from build123d import *

# Parameters (mm, degrees)
BOSS_EXTRUDE2_DEPTH   = 10
BOSS_EXTRUDE2_2_DEPTH = 10
SKETCH4_R             = 2.5
BOSS_EXTRUDE3_DEPTH   = 10
SKETCH8_R             = 22.839298689
CUT_EXTRUDE1_DEPTH    = 10


with BuildPart() as part:
    # Sketch1 → Boss-Extrude2 (new body)
    with BuildSketch(Plane(origin=(0, 0, 0), x_dir=(1, 0, 0), z_dir=(0, 1, 0))):
        Polygon((-26.25, 10.75), (-15, 10.75), (-15, 0), (-23.984756923, -9), (-26.25, -9), (-26.25, -0.114272299), (-29.438415679, -2.555067389), (-29.438415679, 11.073293435), (-26.25, 9.911985917), align=None)
    extrude(amount=BOSS_EXTRUDE2_DEPTH)

    # Sketch8 → Cut-Extrude1 (cut)
    with BuildSketch(Plane(origin=(0, 0, 0), x_dir=(1, 0, 0), z_dir=(0, 1, 0))):
        with Locations((-20.905433381, 4.192616326)):
            Circle(SKETCH8_R)
    extrude(amount=CUT_EXTRUDE1_DEPTH, mode=Mode.SUBTRACT)


with BuildPart() as body_2:
    # Sketch1 → Boss-Extrude2 2 (new body)
    with BuildSketch(Plane(origin=(0, 0, 0), x_dir=(1, 0, 0), z_dir=(0, 1, 0))):
        Polygon((26.25, 10.75), (26.25, 9.911985917), (29.438415679, 11.073293435), (29.438415679, -2.555067389), (26.25, -0.114272299), (26.25, -9), (23.984756923, -9), (15, 0), (15, 10.75), align=None)
    extrude(amount=BOSS_EXTRUDE2_2_DEPTH)

    # Sketch4 → Boss-Extrude3 (add)
    with BuildSketch(Plane(origin=(0, 0, 0), x_dir=(1, 0, 0), z_dir=(0, 1, 0))):
        with BuildLine():
            Line((28.75, -9.5), (33.5, -9.5))
            Line((33.5, -9.5), (33.5, 22.996479512))
            Line((33.5, 22.996479512), (40.345191882, 53.478179684))
            ThreePointArc((40.345191882, 53.478179684), (42.346706654, 60.478565285), (47.83611753, 65.261642557))
            ThreePointArc((47.83611753, 65.261642557), (56.530633029, 70.937419635), (48.815741717, 77.886484122))
            ThreePointArc((48.815741717, 77.886484122), (31.869937483, 69.990732218), (13.180106847, 70.430516322))
            ThreePointArc((13.180106847, 70.430516322), (7.243272391, 73.413222616), (0.765261217, 74.88899747))
            ThreePointArc((0.765261217, 74.88899747), (-7.423605548, 67.770164785), (0.226137573, 60.074922886))
            ThreePointArc((0.226137573, 60.074922886), (22.453224616, 50.257390562), (28.75, 26.78873148))
            Line((28.75, 26.78873148), (28.75, -9.5))
        make_face()
        with Locations(Location((0, 67.5, 0), (0, 0, 270))):
            Circle(SKETCH4_R, mode=Mode.SUBTRACT)
        with Locations(Location((50, 71.444163901, 0), (0, 0, 270))):
            Circle(SKETCH4_R, mode=Mode.SUBTRACT)
    extrude(amount=BOSS_EXTRUDE3_DEPTH)


solid = body_2.part
The model under review builds one solid part; all positions refer to its coordinate system, in mm. A direction names the side the tool comes from. Give positions to 0.01 mm unless a question says otherwise; leave off trailing zeros. Loops run counter-clockwise (first coordinate to the right, second up) from the corner with the lowest first, then second, coordinate; pieces in that order, holes last. Notation, with made-up numbers: (-28, 1.5) -> (-13, 1.5) arc R12 ccw to (-13, 9.5) -> close; hole circle Ø3 at (70.25, -22). An arc over 180 degrees is marked (long way). Put each result on its own line as item: value. Start each with the question number.
1. For faces 5 (the face through (7.33, 4.93, -73.38)), 6 (the face through (26.25, 5, 4)), 7 (the face through (25, 5, 9)), 8 (the face through (33.5, 5, -7)), list the 3-axis set-ups (+Z, -Z, +X, -X, +Y, -Y) from which the entire face can be reached by the end or side of a thin tool; tool diameter is ignored.
2. We need section D-D on z = -2. State the section outline as (x, y) points, then the cut area to 3 significant figures.
3. We need section B-B on z = -67.5. State the section outline as (x, y) points.
4. Clearance check with flat-ended pins moving along their axes: P1, Ø6, axis at x = 41.5, y = 4, coming from the -Z side; P2, Ø4, axis at x = 50, z = -71.44, coming from the -Y side; P3, Ø3, axis at y = 6, z = -16, coming from the -X side; P4, Ø3, axis at y = 4.5, z = -4, coming from the -X side. State where each tip first meets the part, or that it passes through.
5. We need section A-A on x = 50. State the section outline as (y, z) points.
6. Wall thickness on probe 1 along X at (y, z) = (2.25, -14); probe 2 along X at (y, z) = (5.5, -67.5); probe 3 along Z at (x, y) = (18, 2.75): over which ranges is each line inside the solid? List them lowest first.
7. We need section C-C on y = 5.5. State the section outline as (x, z) points, then the cut area to 3 significant figures.
8. Mouldability with a two-part tool opening along Z and no side actions: class faces 1 (the face through (21, 5, -10.75)), 2 (the face through (31, 5, 9.5)), 3 (the face through (0.751, 4.93, -65.115)), 4 (the face through (27, 0, -47)) as released by +Z, released by -Z, zero draft, split by the parting line, or undercut.
Determined:
1. face 5: -Z, +Y, -Y
1. face 6: +Z, +Y, -Y
1. face 7: +Z, -X, +Y, -Y
1. face 8: +Z, +X, +Y, -Y
2. outline: (15, 0) -> (33.5, 0) -> (33.5, 10) -> (15, 10) -> close
2. area: 185 mm^2
3. outline: (-7.43, 0) -> (-2.5, 0) -> (-2.5, 10) -> (-7.43, 10) -> close; (2.5, 0) -> (55.23, 0) -> (55.23, 10) -> (2.5, 10) -> close
4. P1: z = -74.92
4. P2: through
4. P3: x = 28.75
4. P4: x = 15
5. outline: (0, -77.99) -> (10, -77.99) -> (10, -73.94) -> (0, -73.94) -> close; (0, -68.94) -> (10, -68.94) -> (10, -64.89) -> (0, -64.89) -> close
6. probe 1: 28.75 to 33.5
6. probe 2: -7.43 to -2.5, 2.5 to 55.23
6. probe 3: -69.49 to -54.44, -10.75 to 3.01
7. outline: (0.23, -60.07) arc R7.43 ccw (long way) to (0.77, -74.89) arc R27.57 ccw to (13.18, -70.43) arc R41.04 cw to (48.82, -77.89) arc R6.55 ccw (long way) to (47.84, -65.26) arc R12.83 cw to (40.35, -53.48) -> (33.5, -23) -> (33.5, 9.5) -> (28.75, 9.5) -> (28.75, 2.03) -> (26.25, 0.11) -> (26.25, 9) -> (23.98, 9) -> (15, 0) -> (15, -10.75) -> (26.25, -10.75) -> (26.25, -9.91) -> (28.75, -10.82) -> (28.75, -26.79) arc R28.14 cw to start; hole circle Ø5 at (0, -67.5); hole circle Ø5 at (50, -71.44)
7. area: 1,530 mm^2
8. face 1: undercut
8. face 2: released by +Z
8. face 3: undercut
8. face 4: zero draft
